The model under review builds one solid part; all positions refer to its coordinate system, in mm. A direction names the side the tool comes from. Round coordinates to 2 decimals unless told otherwise and drop trailing zeros. Write each loop counter-clockwise with the first axis right and the second up, starting at its lowest first coordinate (ties: lowest second). Pieces come first, ordered by that corner, then holes. Notation, with made-up numbers: (-9.5, 14) -> (20.5, 14) arc R21 cw to (20.5, 44) -> close; hole circle Ø6 at (17, 14). An arc over 180 degrees is marked (long way). Answer in a Markdown table with one row per item. Add a question column.
```python
from build123d import *

# Parameters (mm, degrees)
SKETCH1_W           = 497
SKETCH1_H           = 497
SKETCH1_W_2         = 491
SKETCH1_H_2         = 491
BOSS_EXTRUDE1_DEPTH = 225
SKETCH2_W           = 497
SKETCH2_H           = 497
BOSS_EXTRUDE2_DEPTH = 3
CUT_EXTRUDE1_REACH  = 420.913
SKETCH3_R           = 162.5
SKETCH4_R           = 166
SKETCH4_R_2         = 162.5
BOSS_EXTRUDE3_DEPTH = 40


with BuildPart() as part:
    # Sketch1 → Boss-Extrude1 (new body)
    with BuildSketch(Plane(origin=(0, 0, 0), x_dir=(1, 0, 0), z_dir=(0, 1, 0))):
        Rectangle(SKETCH1_W, SKETCH1_H)
        Rectangle(SKETCH1_W_2, SKETCH1_H_2, mode=Mode.SUBTRACT)
    extrude(amount=BOSS_EXTRUDE1_DEPTH)

    # Sketch2 → Boss-Extrude2 (add)
    with BuildSketch(Plane(origin=(0, 225, 0), x_dir=(1, 0, 0), z_dir=(0, 1, 0))):
        Rectangle(SKETCH2_W, SKETCH2_H)
    extrude(amount=BOSS_EXTRUDE2_DEPTH)

    # Sketch3 → Cut-Extrude1 (cut, up to next)
    with BuildSketch(Plane(origin=(0, 228, 0), x_dir=(1, 0, 0), z_dir=(0, 1, 0)), mode=Mode.PRIVATE) as cut_extrude1_sk1:
        with Locations(Location((0, 0, 0), (0, 0, 270))):
            Circle(SKETCH3_R)
    cut_extrude1_tool1 = extrude(cut_extrude1_sk1.sketch, amount=-CUT_EXTRUDE1_REACH, mode=Mode.PRIVATE) & part.part
    add(cut_extrude1_tool1.solids().sort_by_distance((0, 228, 0))[0], mode=Mode.SUBTRACT)

    # Sketch4 → Boss-Extrude3 (add)
    with BuildSketch(Plane.XZ.offset(-225)):
        with Locations(Location((0, 0, 0), (0, 0, 90))):
            Circle(SKETCH4_R)
        with Locations(Location((0, 0, 0), (0, 0, 90))):
            Circle(SKETCH4_R_2, mode=Mode.SUBTRACT)
    extrude(amount=BOSS_EXTRUDE3_DEPTH)


solid = part.part
```
1. Insertion check: pin 1 Ø4 at (x, z) = (-75.5, 173) entering from -Y; pin 2 Ø1 at (x, z) = (20.5, -161) entering from -Y. Each pin has a flat end and moves straight along its axis. Give the tip position at first contact, or say it passes through.
2. Mouldability with a two-part tool opening along Z and no side actions: class faces 3 (the flat face through (-245.5, 111, 3)), 4 (the flat face through (-3, 228, -169)), 5 (the flat face through (-3, 112, -248.5)) as pulls with the +Z half, pulls with the -Z half, needs draft (parallel to the pull), parting line crosses it, or undercut.
3. Add section A-A on y = 197. Write out the cut boundary in (x, z).
4. Add section D-D on y = 142. Write out the cut boundary in (x, z), plus the area to 3 significant figures.
5. Add section B-B on z = 0. Write out the cut boundary in (x, y).
6. Add section C-C on x = 0. Write out the cut boundary in (y, z).
7. Tool access review of faces 1 (the flat face through (248.5, 112, 3)), 2 (the flat face through (-3, 111, 245.5)): name each direction out of +Z, -Z, +X, -X, +Y, -Y from which nothing blocks a thin tool from reaching the whole face with its end or side.
8. For L1, parallel to X at y = 194, z = 0; L2, parallel to X at y = 53.5, z = -10, list the stretches that pass through material, from the lowest coordinate up.
Filled in:
| question | item | result |
|---|---|---|
| 1 | pin 1 | y = 225 |
| 1 | pin 2 | y = 185 |
| 2 | face 3 | undercut |
| 2 | face 4 | needs draft |
| 2 | face 5 | pulls with the -Z half |
| 3 | outline | (-248.5, -248.5) -> (248.5, -248.5) -> (248.5, 248.5) -> (-248.5, 248.5) -> close; circle Ø332 at (0, 0); hole (-245.5, -245.5) -> (245.5, -245.5) -> (245.5, 245.5) -> (-245.5, 245.5) -> close; hole circle Ø325 at (0, 0) |
| 4 | outline | (-248.5, -248.5) -> (248.5, -248.5) -> (248.5, 248.5) -> (-248.5, 248.5) -> close; hole (-245.5, -245.5) -> (245.5, -245.5) -> (245.5, 245.5) -> (-245.5, 245.5) -> close |
| 4 | area | 5,930 mm² |
| 5 | outline | (-248.5, 0) -> (-245.5, 0) -> (-245.5, 225) -> (-166, 225) -> (-166, 185) -> (-162.5, 185) -> (-162.5, 228) -> (-248.5, 228) -> close; (162.5, 185) -> (166, 185) -> (166, 225) -> (245.5, 225) -> (245.5, 0) -> (248.5, 0) -> (248.5, 228) -> (162.5, 228) -> close |
| 6 | outline | (0, -248.5) -> (228, -248.5) -> (228, -162.5) -> (185, -162.5) -> (185, -166) -> (225, -166) -> (225, -245.5) -> (0, -245.5) -> close; (0, 245.5) -> (225, 245.5) -> (225, 166) -> (185, 166) -> (185, 162.5) -> (228, 162.5) -> (228, 248.5) -> (0, 248.5) -> close |
| 7 | face 1 | +Z, -Z, +X, +Y, -Y |
| 7 | face 2 | -Y |
| 8 | L1 | -248.5 to -245.5, -166 to -162.5, 162.5 to 166, 245.5 to 248.5 |
| 8 | L2 | -248.5 to -245.5, 245.5 to 248.5 |
